```python
from build123d import *

# Parameters (mm, degrees)
SKETCH1_W           = 19.05
SKETCH1_H           = 28.575
SKETCH2_R           = 12.7
BOSS_EXTRUDE1_DEPTH = 695.325
SKETCH3_R           = 12.7
BOSS_EXTRUDE2_DEPTH = 1.374815329
BOSS_EXTRUDE2_TAPER = 30
SKETCH4_R           = 11.90625
BOSS_EXTRUDE3_DEPTH = 11.325184671
CUT_EXTRUDE1_START  = -6.35
CUT_EXTRUDE1_DEPTH  = 6.35
CUT_EXTRUDE2_START  = -6.35
CUT_EXTRUDE2_DEPTH  = 6.35
SKETCH10_R          = 9.525
CUT_EXTRUDE4_DEPTH  = 28.575
SKETCH8_R           = 19.05
BOSS_EXTRUDE5_DEPTH = 114.3
SKETCH9_R           = 19.05
SKETCH9_R_2         = 12.7
CUT_EXTRUDE3_DEPTH  = 114.3


with BuildPart() as part:
    # Sketch1 → Revolve1 (revolve)
    with BuildSketch(Plane.XZ, mode=Mode.PRIVATE) as revolve1_sk:
        with Locations((9.525, -671.5125)):
            Rectangle(SKETCH1_W, SKETCH1_H)
    revolve(revolve1_sk.sketch.rotate(Axis((0, 0, -657.225), (0, 0, -1)), 180), axis=Axis((0, 0, -657.225), (0, 0, -1)))

    # Sketch2 → Boss-Extrude1 (add)
    with BuildSketch(Plane.XY.offset(-657.225)):
        Circle(SKETCH2_R)
    extrude(amount=BOSS_EXTRUDE1_DEPTH)

    # Sketch3 → Boss-Extrude2 (add)
    with BuildSketch(Plane.XY.offset(38.1)):
        Circle(SKETCH3_R)
    extrude(amount=BOSS_EXTRUDE2_DEPTH, taper=BOSS_EXTRUDE2_TAPER)

    # Sketch4 → Boss-Extrude3 (add)
    with BuildSketch(Plane.XY.offset(39.474815329)):
        Circle(SKETCH4_R)
    extrude(amount=BOSS_EXTRUDE3_DEPTH)

    # Sketch5 → Cut-Extrude1 (cut)
    with BuildSketch(Plane.XY.offset(50.8).offset(CUT_EXTRUDE1_START)):
        with BuildLine():
            Line((11.1125, 4.274474566), (11.1125, -4.274474566))
            ThreePointArc((11.1125, -4.274474566), (11.90625, 0), (11.1125, 4.274474566))
        make_face()
    extrude(amount=CUT_EXTRUDE1_DEPTH, mode=Mode.SUBTRACT)

    # Sketch6 → Cut-Extrude2 (cut)
    with BuildSketch(Plane.XY.offset(50.8).offset(CUT_EXTRUDE2_START)):
        with BuildLine():
            Line((-11.1125, -4.274474566), (-11.1125, 4.274474566))
            ThreePointArc((-11.1125, 4.274474566), (-11.90625, 0), (-11.1125, -4.274474566))
        make_face()
    extrude(amount=CUT_EXTRUDE2_DEPTH, mode=Mode.SUBTRACT)

    # Sketch10 → Cut-Extrude4 (cut)
    with BuildSketch(Plane.XY.offset(50.8)):
        Circle(SKETCH10_R)
    extrude(amount=-CUT_EXTRUDE4_DEPTH, mode=Mode.SUBTRACT)

    # Sketch8 → Boss-Extrude5 (add)
    with BuildSketch(Plane(origin=(0, 0, -685.8), x_dir=(-1, 0, 0), z_dir=(0, 0, -1))):
        Circle(SKETCH8_R)
    extrude(amount=BOSS_EXTRUDE5_DEPTH)

    # Sketch9 → Cut-Extrude3 (cut)
    with BuildSketch(Plane.XY.offset(-657.225)):
        with Locations(Location((0, 0, 0), (0, 0, 180))):
            Circle(SKETCH9_R)
        Circle(SKETCH9_R_2, mode=Mode.SUBTRACT)
    extrude(amount=-CUT_EXTRUDE3_DEPTH, mode=Mode.SUBTRACT)


solid = part.part
```
Geometry: final body of the model. Coordinates: model frame, mm. A direction names the side the tool comes from. Give positions to 0.01 mm unless a question says otherwise; leave off trailing zeros. Loops run counter-clockwise (first coordinate to the right, second up) from the corner with the lowest first, then second, coordinate; pieces in that order, holes last. Notation, with made-up numbers: (81.25, -35) -> (94.25, -35) arc R21 ccw to (94.25, -18) -> close; hole circle Ø11 at (18, 33). An arc over 180 degrees is marked (long way). Use one line per item in the form item = value.
Item 1: Access query for faces 4 (the face through (7, -7, 50.8)), 5 (the face through (-4, 12.4, -771.525)). Directions: +Z, -Z, +X, -X, +Y, -Y. A direction counts if a zero-diameter tool reaches every point of the face in a straight line with its end or side. Return the directions, or none.
A:
face_4 = +Z, +X, -X, +Y, -Y
face_5 = +Z
Item 2: Section query A-A on x = 0. Output: boundary loops of the cut face in (y, z) (3 decimals), and give its area (3 significant figures).
A:
outline = (-19.05, -800.1) -> (19.05, -800.1) -> (19.05, -771.525) -> (12.7, -771.525) -> (12.7, 38.1) -> (11.906, 39.475) -> (11.906, 50.8) -> (9.525, 50.8) -> (9.525, 22.225) -> (-9.525, 22.225) -> (-9.525, 50.8) -> (-11.906, 50.8) -> (-11.906, 39.475) -> (-12.7, 38.1) -> (-12.7, -771.525) -> (-19.05, -771.525) -> close
area = 21,400 mm^2
Item 3: Draft query along Y for faces 1 (the face through (0, 0, 22.225)), 2 (the face through (0, 0, -800.1)), 3 (the face through (5.494, -10.563, 45.058)). Return one class per face: pulls with the +Y half, pulls with the -Y half, needs draft (parallel to the pull), parting line crosses it, or undercut.
A:
face_1 = undercut
face_2 = needs draft
face_3 = parting line crosses it
Item 4: Section query B-B on z = -51.5. Output: boundary loops of the cut face in (x, y), and give its area (3 significant figures).
A:
outline = circle Ø25.4 at (0, 0)
area = 507 mm^2
Item 5: Line query: probe 1 along Y at (x, z) = (0, 35.75) (3 decimals); probe 2 along Y at (x, z) = (0, 40) (3 decimals); probe 3 along Z at (x, y) = (-11, -11) (3 decimals). Output: solid intervals per line, ascending.
A:
probe_1 = -12.7 to -9.525, 9.525 to 12.7
probe_2 = -11.906 to -9.525, 9.525 to 11.906
probe_3 = -800.1 to -771.525
Item 6: Pin query (flat end, axial travel): P1, Ø0.9, axis at x = 11.5, y = -1, coming from the +Z side; P2, Ø6, axis at x = -6.5, z = -162.5, coming from the +Y side; P3, Ø8, axis at y = -12.5, z = -125, coming from the -X side; P4, Ø7, axis at y = 2, z = 48, coming from the +X side. Return the tip coordinate at first contact, or that it passes through.
A:
P1 = 50.8
P2 = 12.21
P3 = -9.44
P4 = 11.11
